For this review, use the dimensioned drawing (mm, ordinates from the lowest corner) and the shaded views. Give positions to 0.01 mm unless a question says otherwise; leave off trailing zeros. Write each loop counter-clockwise with the first axis right and the second up, starting at its lowest first coordinate (ties: lowest second). Pieces come first, ordered by that corner, then holes. Notation, with made-up numbers: (11, 62.5) -> (58, 62.5) arc R5 ccw to (58, 69.5) -> close; hole circle Ø8 at (10, 77.5). An arc over 180 degrees is marked (long way). Write each question's results on one line, items separated by ' | '. Start each with the question number.
(1) Take a section at B-B (z = 3.35). State the section outline as (x, y) points.
(2) Take a section at C-C (x = 6.5). State the section outline as (y, z) points, plus the area to 3 significant figures.
(3) Take a section at A-A (y = 0.85). State the section outline as (x, z) points.
(4) Mouldability with a two-part tool opening along X and no side actions: class the marked faces 1 and 2 as released by +X, released by -X, zero draft, split by the parting line, or undercut.
(5) To check wall thickness, follow probe 1 along Y at (x, z) = (9.75, 2.5); probe 2 along Z at (x, y) = (6.25, 0.65); probe 3 along X at (y, z) = (0.65, 2.3). State the ranges of each line that lie inside material, in increasing order.
(6) Take a section at D-D (y = 0.25). State the section outline as (x, z) points (1 decimal).
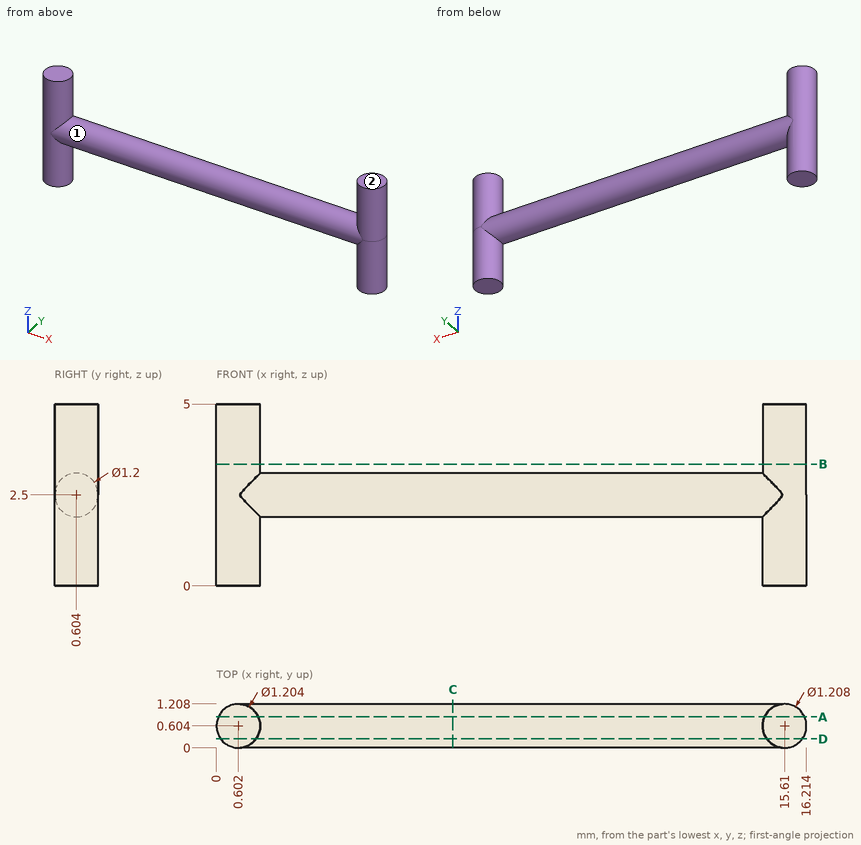
Report:
1) outline: circle Ø1.2 at (0.6, 0.6); circle Ø1.21 at (15.61, 0.6)
2) outline: circle Ø1.2 at (0.6, 2.5) | area: 1.13 mm2
3) outline: (0.05, 0) -> (1.15, 0) -> (1.15, 1.95) -> (15.06, 1.95) -> (15.06, 0) -> (16.16, 0) -> (16.16, 5) -> (15.06, 5) -> (15.06, 3.05) -> (1.15, 3.05) -> (1.15, 5) -> (0.05, 5) -> close
4) face 1: undercut | face 2: zero draft
5) probe 1: 0 to 1.2 | probe 2: 1.9 to 3.1 | probe 3: 0 to 16.21
6) outline: (0.1, 0) -> (1.1, 0) -> (1.1, 2) -> (15.1, 2) -> (15.1, 0) -> (16.1, 0) -> (16.1, 5) -> (15.1, 5) -> (15.1, 3) -> (1.1, 3) -> (1.1, 5) -> (0.1, 5) -> close
